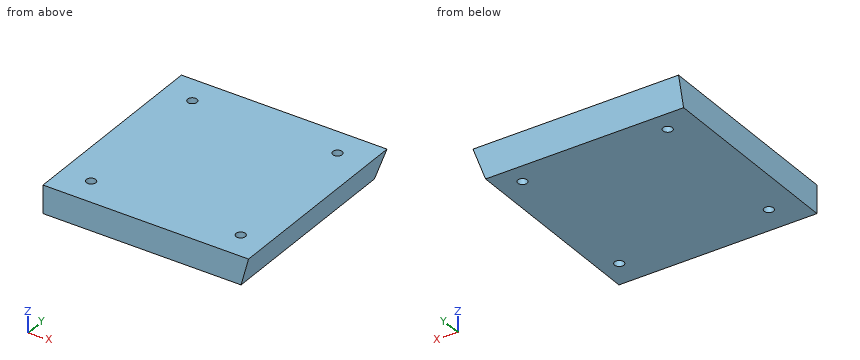
from build123d import *

# Parameters (mm, degrees)
F0_W     = 139.7
F0_H     = 139.7
F0_R     = 3.175
F1_DEPTH = 19.05
F2_SIZE2 = 5.104422
F2_SIZE  = 19.04999


# Not quite as in the source:
# - a fillet or chamfer is up to 0.001 mm smaller than in the source, because OpenCascade refuses the exact size


with BuildPart() as f1:
    # F0 (on Top) → F1 (new body)
    with BuildSketch(Plane.XY):
        with Locations((-3.4590801224, 34.0288509236)):
            Rectangle(F0_W, F0_H)
        with Locations((-53.1284622848, -17.2076094896)):
            Circle(F0_R, mode=Mode.SUBTRACT)
        with Locations((48.5374927521, -17.2076094896)):
            Circle(F0_R, mode=Mode.SUBTRACT)
        with Locations((-53.1284622848, 84.8837196827)):
            Circle(F0_R, mode=Mode.SUBTRACT)
        with Locations((45.559823513, 84.8837196827)):
            Circle(F0_R, mode=Mode.SUBTRACT)
    extrude(amount=F1_DEPTH)

    # F2 (size 19.05 and 5.1044321158 in the source; OpenCascade refuses exactly that, so slightly less here)
    f2_edges = [f1.edges().sort_by_distance(p)[0] for p in [
        (66.39092, 34.028851, 0),
        (-3.45908, 103.878851, 0),
    ]]
    chamfer(f2_edges, length=F2_SIZE, length2=F2_SIZE2)


solid = f1.part
Source: CAD feature listing. Evaluate the final solid. Frame: model axes, mm. Round coordinates to 2 decimals unless told otherwise and drop trailing zeros. One line per item, written item: value. Start each with the question number.
Item 1: Section query A-A (z = 11). State how many separate pieces and enclosed holes the cut face has, plus the area to 3 significant figures.
Item 2: Ray query, L1, parallel to X at y = 85, z = 17.5; L2, parallel to Y at x = 50, z = 5.25; L3, parallel to X at y = 75, z = 17.5. Return the intervals inside material, ascending. Write a range as from..to.
Item 3: Pin query (flat end, axial travel): pin 1 (5 mm diameter, centred on y = 1.5, z = 7.5, fed in from +X). Return the tip coordinate at first contact, or that it passes through.
Result set:
1. separate pieces: 1
1. enclosed holes: 4
1. area: 18,800 mm²
2. L1: x = -73.31..-56.3, -49.96..42.39, 48.73..65.98
2. L2: y = -35.82..-20.03, -14.39..100.18
2. L3: x = -73.31..65.98
3. pin 1: stops at x = 63.97
